from build123d import *

# Parameters (mm, degrees)
SKETCH2_R          = 3
CUT_EXTRUDE1_DEPTH = 10
SKETCH3_R          = 1.5
CUT_EXTRUDE2_DEPTH = 10
CUT_EXTRUDE3_DEPTH = 2.2
SKETCH6_W          = 24
SKETCH6_H          = 3.713708499
CUT_EXTRUDE4_DEPTH = 8


with BuildPart() as part:
    # Sketch1 → Revolve1 (revolve)
    with BuildSketch(Plane.XY, mode=Mode.PRIVATE) as revolve1_sk:
        Polygon((-45.933362566, 0), (38.066637434, 0), (38.066637434, 6), (27.066637434, 6), (27.066637434, 5), (26.066637434, 5), (26.066637434, 6), (-17.933362566, 6), (-17.933362566, 5), (-18.933362566, 5), (-18.933362566, 6), (-45.933362566, 6), align=None)
    revolve(revolve1_sk.sketch.rotate(Axis((-45.933362566, 0, 0), (1, 0, 0)), 90), axis=Axis((-45.933362566, 0, 0), (1, 0, 0)))

    # Sketch2 → Cut-Extrude1 (cut)
    with BuildSketch(Plane(origin=(38.066637434, 0, 0), x_dir=(0, 0, -1), z_dir=(1, 0, 0))):
        Circle(SKETCH2_R)
    extrude(amount=-CUT_EXTRUDE1_DEPTH, mode=Mode.SUBTRACT)

    # Sketch3 → Cut-Extrude2 (cut)
    with BuildSketch(Plane.XY):
        with Locations((34.231149576, 0)):
            Circle(SKETCH3_R)
    extrude(amount=-CUT_EXTRUDE2_DEPTH, mode=Mode.SUBTRACT)

    # Sketch5 → Cut-Extrude3 (cut)
    with BuildSketch(Plane(origin=(0, 6, 0), x_dir=(1, 0, 0), z_dir=(0, 1, 0))):
        with BuildLine():
            Line((-5.933362566, 2), (14.066637434, 2))
            ThreePointArc((14.066637434, 2), (16.066637434, 0), (14.066637434, -2))
            Line((14.066637434, -2), (-5.933362566, -2))
            ThreePointArc((-5.933362566, -2), (-7.933362566, 0), (-5.933362566, 2))
        make_face()
    extrude(amount=-CUT_EXTRUDE3_DEPTH, mode=Mode.SUBTRACT)

    # Sketch6 → Cut-Extrude4 (cut, symmetric)
    with BuildSketch(Plane.XY):
        with Locations((4.066637434, 5.65685425)):
            Rectangle(SKETCH6_W, SKETCH6_H)
    extrude(amount=CUT_EXTRUDE4_DEPTH, both=True, mode=Mode.SUBTRACT)


solid = part.part
Source: CAD feature listing. Evaluate the final solid. Frame: model axes, mm. A direction names the side the tool comes from. Coordinates: 2 decimals unless noted, no trailing zeros. Loops run counter-clockwise (first coordinate to the right, second up) from the corner with the lowest first, then second, coordinate; pieces in that order, holes last. Notation, with made-up numbers: M -37.75,19.5 L -19.75,19.5 A20 ccw -19.75,41.5 Z; hole C -34.75,81.25 d7. An arc over 180 degrees is marked long. Answer in a Markdown table with one row per item.
Q1. Draft query along Y for faces 6 (the cylindrical face through (33, 0, 3)), 7 (the cylindrical face through (3.76, -5.95, -0.78)), 8 (the flat face through (27.067, -4, -4)). Return one class per face: pulls with the +Y half, pulls with the -Y half, needs draft (parallel to the pull), parting line crosses it, or undercut.
Answers below:
| item | result |
|---|---|
| face 6 | undercut |
| face 7 | parting line crosses it |
| face 8 | needs draft |
Q2. Section D-D on x = -1.5. Return the cut outline in (y, z).
Answers below:
| item | result |
|---|---|
| outline | M 3.8,-4.64 L 3.8,4.64 A6 ccw long Z |
Q3. Section C-C on x = -10. Return the cut outline in (y, z), plus the area to 3 significant figures.
Answers below:
| item | result |
|---|---|
| outline | C 0,0 d12 |
| area | 113 mm^2 |
Q4. Section A-A on y = 0. Return the cut outline in (x, z), plus the area to 3 significant figures.
Answers below:
| item | result |
|---|---|
| outline | M -45.93,-6 L -18.93,-6 L -18.93,-5 L -17.93,-5 L -17.93,-6 L 26.07,-6 L 26.07,-5 L 27.07,-5 L 27.07,-6 L 32.73,-6 L 32.73,-3 L 28.07,-3 L 28.07,3 L 38.07,3 L 38.07,6 L 27.07,6 L 27.07,5 L 26.07,5 L 26.07,6 L -17.93,6 L -17.93,5 L -18.93,5 L -18.93,6 L -45.93,6 Z; M 35.73,-6 L 38.07,-6 L 38.07,-3 L 35.73,-3 Z |
| area | 935 mm^2 |
Q5. Set-up query: faces 1 (the flat face through (16.067, 5, 0)), 2 (the flat face through (-18.933, -4, 4)), 3 (the cylindrical face through (32.49, -1.802, 5.723)), 4 (the flat face through (28.067, 0, 0)), 5 (the cylindrical face through (35.66, 0.45, -4.28)). Return all of +Z, -Z, +X, -X, +Y, -Y with unobstructed straight access to the full face (end or side cutting, diameter ignored); none if empty.
Answers below:
| item | result |
|---|---|
| face 1 | +Z, -Z, +Y |
| face 2 | none |
| face 3 | +X, -X |
| face 4 | +X |
| face 5 | -Z |
Q6. First-contact query: pin 1 (6 mm diameter, centred on y = -1.5, z = -2.5, fed in from +X); pin 2 (1.8 mm diameter, centred on y = 0, z = -0.5, fed in from +X); pin 3 (3 mm diameter, centred on x = 3.5, y = 4.5, fed in from +Z); pin 4 (3 mm diameter, centred on x = -37, y = -2.5, fed in from +Z). Flat tips, straight axial feed; report the tip coordinate or a pass-through.
Answers below:
| item | result |
|---|---|
| pin 1 | stops at x = 38.07 |
| pin 2 | stops at x = 28.07 |
| pin 3 | stops at z = 5.2 |
| pin 4 | stops at z = 5.92 |
Q7. Section B-B on z = 0. Return the cut outline in (x, y), plus the area to 3 significant figures.
Answers below:
| item | result |
|---|---|
| outline | M -45.93,-6 L -18.93,-6 L -18.93,-5 L -17.93,-5 L -17.93,-6 L 26.07,-6 L 26.07,-5 L 27.07,-5 L 27.07,-6 L 38.07,-6 L 38.07,-3 L 28.07,-3 L 28.07,3 L 38.07,3 L 38.07,6 L 27.07,6 L 27.07,5 L 26.07,5 L 26.07,6 L 16.07,6 L 16.07,3.8 L -7.93,3.8 L -7.93,6 L -17.93,6 L -17.93,5 L -18.93,5 L -18.93,6 L -45.93,6 Z |
| area | 891 mm^2 |
Q8. Ray query, probe 1 along X at (y, z) = (-3, 5); probe 2 along X at (y, z) = (0, -5.3); probe 3 along X at (y, z) = (5.75, 1). Return the intervals inside material, ascending. Write a range as from..to.
Answers below:
| item | result |
|---|---|
| probe 1 | x = -45.93..-18.93, -17.93..26.07, 27.07..38.07 |
| probe 2 | x = -45.93..-18.93, -17.93..26.07, 27.07..32.73, 35.73..38.07 |
| probe 3 | x = -45.93..-18.93, -17.93..-7.93, 16.07..26.07, 27.07..38.07 |
